Autodesk Fusion 360 part; units mm, degrees
sketch "Sketch1" plane through (0, 0, 0) normal (0, 0, 1) x (1, 0, 0)
  line L0 (36.5, 30.5) -> (-32.5, 30.5)
  line L1 (-32.5, 30.5) -> (-32.5, -30.5)
  line L2 (-32.5, -30.5) -> (36.5, -30.5)
  line L3 (36.5, -30.5) -> (36.5, 30.5)
  line L4 (36.5, -27.25) -> (-32.5, -27.25)
  line L5 (-32.5, -27.25) -> (-32.5, 27.25)
  line L6 (-32.5, 27.25) -> (36.5, 27.25)
  line L7 (36.5, 27.25) -> (36.5, -27.25)
  line L8 (33, 35.5) -> (-32.5, 35.5)
  line L9 (-32.5, 35.5) -> (-32.5, 30.5)
  line L10 (1.75, 0) -> (22.5, 0)
  line L11 (-32.5, -35.5) -> (-32.5, -30.5)
  line L12 (32.9935, -35.55) -> (-32.5, -35.5)
  line L13 (41.5, -27.05) -> (41.5, 27)
  arc A0 (32.9935, -35.55) -> (41.5, -27.05) centre (33, -27.05) ccw
  arc A1 (41.5, 27) -> (33, 35.5) centre (33, 27) ccw
  dimension "d1" = 69
  dimension "d2" = 61
  dimension "d3" = 69
  dimension "d4" = 54.5
  dimension "d46" = 8.5
extrude "Extrude1" add sketch "Sketch1" along normal blind 6.45 contours L0 L1 L3 L6 | L0 L2 L3 L7 L8 L9 L11 L12 L13 A0 A1 | L1 L2 L3 L4
extrude "Extrude2" add sketch "Sketch1" along normal blind 22 contours L0 L2 L3 L7 L8 L9 L11 L12 L13 A0 A1
extrude "Extrude3" add sketch "Sketch1" along normal blind 23 and the other way blind -20
sketch "Sketch2" plane through (0, 0, 23) normal (0, 0, 1) x (-1, 0, 0)
  line L0 (-33, -35.5) -> (32.5, -35.5)
  line L1 (32.5, -35.5) -> (32.5, 35.5)
  line L2 (32.5, 35.5) -> (-32.9935, 35.55)
  circle A0 centre (20, 0) radius 1.75
  circle A1 centre (-15, 0) radius 1.75
  arc A2 (-32.9935, 35.55) -> (-41.5, 27.05) centre (-33, 27.05) ccw
  line L3 (-41.5, 27.05) -> (-41.5, -27)
  arc A3 (-41.5, -27) -> (-33, -35.5) centre (-33, -27) ccw
  dimension "d33" = 3.5
  dimension "d34" = 3.5
extrude "Extrude4" cut sketch "Sketch2" against normal blind 5 contours A0 | A1
sketch "Sketch3" plane through (0, 35.5, 0) normal (0, 1, 0) x (-1, 0, 0)
  line L0 (-33, 0) -> (32.5, 0)
  line L1 (32.5, 0) -> (32.5, 23)
  line L2 (32.5, 23) -> (-33, 23)
  line L3 (32.5, 23) -> (34.5, 23)
  line L4 (34.5, 23) -> (34.5, 0)
  line L5 (34.5, 0) -> (32.5, 0)
  line L6 (34.5, 0) -> (34.5, 8)
  line L7 (34.5, 23) -> (46.0025, 23)
  line L8 (34.5, 0) -> (46.0025, 23)
  line L9 (-33, 23) -> (-33, 0)
  dimension "d47" = 26.57
extrude "Extrude5" add sketch "Sketch3" against normal blind 5 contours L1 L3 L4 L5 L6 | L4 L6 L7 L8
extrude "Extrude6" add sketch "Sketch3" along normal blind -71 and the other way blind 66 contours L1 L3 L4 L5 L6 | L4 L6 L7 L8
sketch "Sketch4" plane through (0, 30.5, 0) normal (0, -1, 0) x (1, 0, 0)
  line L0 (-32.5, 20) -> (-32.5, 23)
  line L1 (-32.5, 23) -> (-46.0025, 23)
  line L2 (-46.0025, 23) -> (-34.5, 0)
  line L3 (-34.5, 0) -> (-37.7235, 6.4455)
  line L4 (-32.5, 6.4455) -> (-37.7235, 6.4455)
  line L5 (-32.5, 6.4455) -> (-32.5, 0)
  line L6 (-34.5, 0) -> (-32.5, 0)
  line L7 (36.5, 20) -> (-32.5, 20)
  line L8 (-32.5, 6.45) -> (36.5, 6.45)
  line L9 (36.5, 6.45) -> (36.5, 20)
extrude "Extrude7" add sketch "Sketch4" along normal blind 3.25
extrude "Extrude8" add sketch "Sketch4" along normal blind 61 and the other way blind -57.75
chamfer "Chamfer2" distance 1 angle 45 2 edges at (-18.3684, 0.6328, 20) (16.6316, 0.6328, 20)
sketch "Sketch5" plane through (0, 30.5, 0) normal (0, -1, 0) x (1, 0, 0)
  line L0 (-37.7235, 6.4455) -> (-32.5, 6.4455)
  line L1 (-32.5, 6.4455) -> (-32.5, 6.45)
  line L2 (-46.0025, 23) -> (-37.7235, 6.4455)
  line L3 (-32.5, 6.45) -> (36.5, 6.45)
  line L4 (36.5, 6.45) -> (36.5, 20)
  line L5 (36.5, 20) -> (-32.5, 20)
  line L6 (-46.0025, 23) -> (-27, 23)
  line L7 (-29, 20) -> (-51.5326, 20)
  line L8 (-43.3815, 17.7592) -> (-46.4301, 23.8551)
  line L9 (-28, 19) -> (-27.5232, 25.3132)
extrude "Extrude9" add sketch "Sketch5" along normal blind 61 contours L2 L5 L6 L7 L8 L9
sketch "Sketch6" plane through (0, 0, 20) normal (0, 0, -1) x (1, 0, 0)
  circle A0 centre (-20, 0) radius 2.75
  line L0 (36.5, 30.5) -> (-44.5022, 30.5)
  line L1 (-44.5022, -30.5) -> (36.5, -30.5)
  line L2 (36.5, -30.5) -> (36.5, 30.5)
  circle A1 centre (15, 0) radius 2.75
  line L3 (15, -11) -> (-20, -11)
  arc A2 (-20, -11) -> (-20, -19) centre (-20, -15) ccw
  line L4 (-20, -19) -> (15, -19)
  arc A3 (15, -19) -> (15, -11) centre (15, -15) ccw
  line L5 (15, -15) -> (-20, -15) construction
  line L6 (1.75, 0) -> (22.5, 0)
  line L7 (-20, 19) -> (15, 19)
  arc A4 (15, 11) -> (15, 19) centre (15, 15) ccw
  line L8 (15, 11) -> (-20, 11)
  arc A5 (-20, 19) -> (-20, 11) centre (-20, 15) ccw
  line L9 (-44.5022, 30.5) -> (-44.5022, -30.5)
extrude "Extrude10" cut sketch "Sketch6" against normal blind 25 contours L3 A2 L4 A3 | L7 A4 L8 A5
Could you check a few things on this model? Use its own coordinates, in mm. A direction names the side the tool comes from. Give positions to 0.01 mm unless a question says otherwise; leave off trailing zeros. Order: outer loops, then holes, each group sorted by start corner. A loop starts at its lowest first (then second) coordinate and runs counter-clockwise, first axis right, second up.
Item 1: For faces 4 (the face through (38.94, 33.08, 11.34)), 5 (the face through (2, 29, 6.45)), 6 (the face through (-2, 11, 21)), which set-ups out of +Z, -Z, +X, -X, +Y, -Y let a thin tool reach every point of the face, with its end or its side?
Item 2: If we mould it in two halves opening along Z, with no side actions, what happens to faces 1 (the face through (37, -2, 0)), 2 (the face through (-18.25, -0.08, 22.01)), 3 (the face through (-5, -30.5, 13))? For each: pulls with the +Z half, pulls with the -Z half, needs draft (parallel to the pull), parting line crosses it, or undercut.
Item 3: If we section it at A-A, the plane y = -15: Write out the boundary of the cut face in (x, z).
Item 4: If we section it at D-D, the plane z = 10.5: Write out the boundary of the cut face in (x, y), plus the area to 3 significant figures.
Item 5: If we section it at B-B, the plane x = -10: Write out the boundary of the cut face in (y, z), plus the area to 3 significant figures.
Item 6: If we section it at C-C, the plane y = 0: Write out the boundary of the cut face in (x, z), plus the area to 3 significant figures.
Item 7: I'm going to push flat-ended pins straight in: pin 1 (2 mm diameter, centred on x = -20, y = 0, fed in from +Z); pin 2 (8 mm diameter, centred on y = -17.5, z = 17, fed in from -X); pin 3 (18.5 mm diameter, centred on x = 10.5, y = -6, fed in from -Z); pin 4 (4 mm diameter, centred on y = -11, z = 12.5, fed in from -X). Where does each tip first touch, or does it pass through?
Item 8: I need wall thicknesses on line 1 (Y direction, x = 15, z = 21.9); line 2 (Y direction, x = 16, z = 21.25); line 3 (X direction, y = 0, z = 21.7). Which ranges of each line are inside material? Lowest first, please.
Values:
1. face 4: +Z, -Z, +X, +Y
1. face 5: -X
1. face 6: +Z, -Z
2. face 1: pulls with the -Z half
2. face 2: needs draft
2. face 3: undercut
3. outline: (-46, 23) - (-44.5, 20) - (-24, 20) - (-24, 23) - close; (19, 20) - (36.5, 20) - (36.5, 0) - (41.5, 0) - (41.5, 23) - (19, 23) - close
4. outline: (-39.75, -35.5) - (-32.5, -35.5) - (32.99, -35.55) arc R8.5 ccw to (41.5, -27.05) - (41.5, 27) arc R8.5 ccw to (33, 35.5) - (-39.75, 35.5) - (-39.75, 30.5) - (36.5, 30.5) - (36.5, -30.5) - (-39.75, -30.5) - close
4. area: 1,090 mm2
5. outline: (-35.52, 0) - (-27.25, 0) - (-27.25, 6.45) - (-30.5, 6.45) - (-30.5, 20) - (-19, 20) - (-19, 23) - (-35.52, 23) - close; (-11, 20) - (11, 20) - (11, 23) - (-11, 23) - close; (19, 20) - (30.5, 20) - (30.5, 6.45) - (27.25, 6.45) - (27.25, 0) - (35.5, 0) - (35.5, 23) - (19, 23) - close
5. area: 407 mm2
6. outline: (-46, 23) - (-44.5, 20) - (-22.75, 20) - (-21.75, 21) - (-21.75, 23) - close; (-18.25, 21) - (-17.25, 20) - (12.25, 20) - (13.25, 21) - (13.25, 23) - (-18.25, 23) - close; (16.75, 21) - (17.75, 20) - (36.5, 20) - (36.5, 0) - (41.5, 0) - (41.5, 23) - (16.75, 23) - close
6. area: 337 mm2
7. pin 1: passes through
7. pin 2: stops at x = -45
7. pin 3: stops at z = 20
7. pin 4: stops at x = 36.5
8. line 1: y = -35.54 to -19, -11 to -1.75, 1.75 to 11, 19 to 35.5
8. line 2: y = -35.54 to -18.87, -11.13 to -1.44, 1.44 to 11.13, 18.87 to 35.5
8. line 3: x = -45.35 to -21.75, -18.25 to 13.25, 16.75 to 41.5
